from build123d import *

# Parameters (mm, degrees)
SKETCH2_W           = 66.16954
SKETCH2_H           = 33.1978
BOSS_EXTRUDE1_DEPTH = 96.901
FILLET1_R           = 0.5
SKETCH3_W           = 0.889
SKETCH3_H           = 6.1214
CIRPATTERN1_COUNT   = 2


with BuildPart() as part:
    # Sketch2 → Boss-Extrude1 (new body)
    with BuildSketch(Plane(origin=(0, 0, 0), x_dir=(1, 0, 0), z_dir=(0, 1, 0))):
        Rectangle(SKETCH2_W, SKETCH2_H)
    extrude(amount=BOSS_EXTRUDE1_DEPTH)

    # Fillet1
    fillet1_edges = [part.edges().sort_by_distance(p)[0] for p in [
        (-33.08477, 96.901, 0),
        (0, 96.901, 16.5989),
        (33.08477, 96.901, 0),
        (0, 0, 16.5989),
        (-33.08477, 0, 0),
        (0, 0, -16.5989),
        (33.08477, 0, 0),
        (33.08477, 48.4505, 16.5989),
        (-33.08477, 48.4505, 16.5989),
        (-33.08477, 48.4505, -16.5989),
        (33.08477, 48.4505, -16.5989),
        (0, 96.901, -16.5989),
    ]]
    fillet(fillet1_edges, radius=FILLET1_R)

    # Sweep1: sweep along a path in Sketch4
    with BuildLine(Plane(origin=(0, 0, -16.5989), x_dir=(-1, 0, 0), z_dir=(0, 0, -1))) as sweep1_path:
        Line((23.25497, 96.901), (23.25497, 99.4824))
        ThreePointArc((23.25497, 99.4824), (22.962076781, 100.189506781), (22.25497, 100.4824))
        Line((22.25497, 100.4824), (14.63497, 100.4824))
    # Sketch3 → Sweep1 (sweep)
    with BuildSketch(Plane(origin=(0, 96.901, 0), x_dir=(1, 0, 0), z_dir=(0, 1, 0))):
        with Locations((-22.81047, 12.2532)):
            Rectangle(SKETCH3_W, SKETCH3_H)
    sweep1 = sweep(path=sweep1_path.line)

    # CirPattern1: Sweep1 ×2 about axis
    cirpattern1_axis = Axis((0, 0, 0), (0, 1, 0))
    for i in range(1, CIRPATTERN1_COUNT):
        add(sweep1.rotate(cirpattern1_axis, i * 360 / CIRPATTERN1_COUNT))


solid = part.part
Here's how the part is built. I have some questions about the finished solid (model axes, mm). A direction names the side the tool comes from. Round coordinates to 2 decimals unless told otherwise and drop trailing zeros. Loops run counter-clockwise (first coordinate to the right, second up) from the corner with the lowest first, then second, coordinate; pieces in that order, holes last. Notation, with made-up numbers: (-12, 30.25) -> (32, 30.25) arc R26 ccw to (32, 66.25) -> close; hole circle Ø10 at (28, 41.25). An arc over 180 degrees is marked (long way). Write each question's results on one line, items separated by ' | '.
(1) If we section it at C-C, the plane z = 13.5: List the corners of the cut face in (x, y) for me.
Worked answers:
outline: (-33.08, 0.5) arc R0.5 ccw to (-32.58, 0) -> (32.58, 0) arc R0.5 ccw to (33.08, 0.5) -> (33.08, 96.4) arc R0.5 ccw to (32.58, 96.9) -> (23.25, 96.9) -> (23.25, 99.48) arc R1 ccw to (22.25, 100.48) -> (14.63, 100.48) -> (14.63, 99.59) -> (22.25, 99.59) arc R0.11 cw to (22.37, 99.48) -> (22.37, 96.9) -> (-32.58, 96.9) arc R0.5 ccw to (-33.08, 96.4) -> close
(2) If we section it at A-A, the plane z = -0.5: List the corners of the cut face in (x, y) for me.
Worked answers:
outline: (-33.08, 0.5) arc R0.5 ccw to (-32.58, 0) -> (32.58, 0) arc R0.5 ccw to (33.08, 0.5) -> (33.08, 96.4) arc R0.5 ccw to (32.58, 96.9) -> (-32.58, 96.9) arc R0.5 ccw to (-33.08, 96.4) -> close
(3) For P1, Ø1.1, axis at x = -20.5, y = 98.5, coming from the -Z side; P2, Ø10, axis at x = -2.5, z = -7.5, coming from the +Y side; P3, Ø1, axis at y = 100, z = 12, coming from the -X side; P4, Ø2, axis at y = 98, z = -11.5, coming from the -X side (3 decimals), each with a flat end and sliding along its axis, tell me the tip position at first contact or that it passes through.
Worked answers:
P1: through | P2: y = 96.9 | P3: x = 14.63 | P4: x = -23.255
(4) For faces 1 (the face through (23.255, 98, 12)), 2 (the face through (18, 99.593, 12)), 3 (the face through (20, 100, 15.314)), 4 (the face through (-22.366, 98, -12)), 5 (the face through (20, 100, 9.193)), which set-ups out of +Z, -Z, +X, -X, +Y, -Y let a thin tool reach every point of the face, with its end or its side?
Worked answers:
face 1: +Z, -Z, +X, +Y | face 2: +Z, -Z, -X | face 3: +Z, +X, -X, +Y | face 4: +Z, -Z, +X | face 5: -Z, +X, -X, +Y
(5) If I drill on L1, parallel to Y at x = 15, z = 10.5; L2, parallel to Y at x = 12.5, z = -5, over which ranges is the centre line in solid material (lowest first)?
Worked answers:
L1: 0 to 96.9, 99.59 to 100.48 | L2: 0 to 96.9
(6) We'd pull the mould along Y, two halves only. Please class faces 6 (the face through (-23.255, 98, -12)), 7 (the face through (18, 100.482, 12)), 8 (the face through (0, 0, 0)), 9 (the face through (-18, 99.593, -12)): released by +Y, released by -Y, zero draft, split by the parting line, or undercut.
Worked answers:
face 6: zero draft | face 7: released by +Y | face 8: released by -Y | face 9: undercut
(7) If we section it at B-B, the plane x = 28: List the corners of the cut face in (y, z) for me.
Worked answers:
outline: (0, -16.1) arc R0.5 ccw to (0.5, -16.6) -> (96.4, -16.6) arc R0.5 ccw to (96.9, -16.1) -> (96.9, 16.1) arc R0.5 ccw to (96.4, 16.6) -> (0.5, 16.6) arc R0.5 ccw to (0, 16.1) -> close
